from build123d import *

# Parameters (mm, degrees)
SKETCH_1_W       = 50
SKETCH_1_H       = 100
EXTRUDE_1_DEPTH  = 4
FILLET_2_R       = 5
FILLET_3_R       = 5
FILLET_4_R       = 5
FILLET_5_R       = 5
SKETCH_2_R       = 3
EXTRUDE_2_DEPTH  = 10
SKETCH_3_R       = 3
EXTRUDE_3_DEPTH  = 15
SKETCH_6_W       = 50
SKETCH_6_H       = 100
EXTRUDE_4_DEPTH  = 4
FILLET_6_R       = 5
FILLET_7_R       = 5
FILLET_8_R       = 5
FILLET_9_R       = 5
SKETCH_7_W       = 50
SKETCH_7_H       = 100
EXTRUDE_5_DEPTH  = 4
EXTRUDE_START    = 15
SKETCH_8_R       = 3
EXTRUDE_6_DEPTH  = 15
SKETCH_9_W       = 50
SKETCH_9_H       = 100
EXTRUDE_7_DEPTH  = 4
SKETCH_11_R      = 3
EXTRUDE_9_DEPTH  = 15
FILLET_10_R      = 5
FILLET_11_R      = 5
FILLET_12_R      = 5
FILLET_13_R      = 5
FILLET_14_R      = 5
FILLET_15_R      = 5
FILLET_16_R      = 5
FILLET_17_R      = 5
SKETCH_13_W      = 50
SKETCH_13_H      = 100
EXTRUDE_10_DEPTH = 4
SKETCH_14_R      = 3
EXTRUDE_11_DEPTH = 15
FILLET_18_R      = 5
FILLET_19_R      = 5
FILLET_20_R      = 5
FILLET_21_R      = 5
SKETCH_15_R      = 3
EXTRUDE_12_DEPTH = 10
SHELL_1_T        = -0.5


with BuildPart() as part:
    # Sketch 1 → Extrude 1 (new body)
    with BuildSketch(Plane.XY):
        Rectangle(SKETCH_1_W, SKETCH_1_H)
    extrude(amount=EXTRUDE_1_DEPTH)

    # Fillet 2
    fillet_2_edges = [part.edges().sort_by_distance(p)[0] for p in [
        (25, 50, 2),
    ]]
    fillet(fillet_2_edges, radius=FILLET_2_R)

    # Fillet 3
    fillet_3_edges = [part.edges().sort_by_distance(p)[0] for p in [
        (-25, 50, 2),
    ]]
    fillet(fillet_3_edges, radius=FILLET_3_R)

    # Fillet 4
    fillet_4_edges = [part.edges().sort_by_distance(p)[0] for p in [
        (25, -50, 2),
    ]]
    fillet(fillet_4_edges, radius=FILLET_4_R)

    # Fillet 5
    fillet_5_edges = [part.edges().sort_by_distance(p)[0] for p in [
        (-25, -50, 2),
    ]]
    fillet(fillet_5_edges, radius=FILLET_5_R)

    # Sketch 2 → Extrude 2 (add)
    with BuildSketch(Plane.XY.offset(4)):
        with Locations((20, 45)):
            Circle(SKETCH_2_R)
    extrude(amount=EXTRUDE_2_DEPTH)

    # Sketch 3 → Extrude 3 (add)
    with BuildSketch(Plane(origin=(0, 0, 0), x_dir=(-1, 0, 0), z_dir=(0, 0, -1))):
        with Locations(Location((20, -45, 0), (0, 0, 180))):
            Circle(SKETCH_3_R)
    extrude(amount=EXTRUDE_3_DEPTH)

    # Sketch 6 → Extrude 4 (add)
    with BuildSketch(Plane(origin=(0, 0, -15), x_dir=(-1, 0, 0), z_dir=(0, 0, -1))):
        Rectangle(SKETCH_6_W, SKETCH_6_H)
    extrude(amount=EXTRUDE_4_DEPTH)

    # Fillet 6
    fillet_6_edges = [part.edges().sort_by_distance(p)[0] for p in [
        (25, 50, -17),
    ]]
    fillet(fillet_6_edges, radius=FILLET_6_R)

    # Fillet 7
    fillet_7_edges = [part.edges().sort_by_distance(p)[0] for p in [
        (-25, 50, -17),
    ]]
    fillet(fillet_7_edges, radius=FILLET_7_R)

    # Fillet 8
    fillet_8_edges = [part.edges().sort_by_distance(p)[0] for p in [
        (-25, -50, -17),
    ]]
    fillet(fillet_8_edges, radius=FILLET_8_R)

    # Fillet 9
    fillet_9_edges = [part.edges().sort_by_distance(p)[0] for p in [
        (25, -50, -17),
    ]]
    fillet(fillet_9_edges, radius=FILLET_9_R)



with BuildPart() as body_2:
    # Sketch 7 → Extrude 5 (new body)
    with BuildSketch(Plane(origin=(0, 0, -34), x_dir=(-1, 0, 0), z_dir=(0, 0, -1))):
        Rectangle(SKETCH_7_W, SKETCH_7_H)
    extrude(amount=EXTRUDE_5_DEPTH)


with BuildPart() as part_1:
    add(part.part)

    add(body_2.part)  # Extrude 6 merges body 2
    # Sketch 8 → Extrude 6 (add)
    with BuildSketch(Plane(origin=(0, 0, -19), x_dir=(-1, 0, 0), z_dir=(0, 0, -1)).offset(EXTRUDE_START)):
        with Locations(Location((-20, 45, 0), (0, 0, 180))):
            Circle(SKETCH_8_R)
    extrude(amount=-EXTRUDE_6_DEPTH)



with BuildPart() as body_2_2:
    # Sketch 9 → Extrude 7 (new body)
    with BuildSketch(Plane(origin=(0, 0, -53), x_dir=(-1, 0, 0), z_dir=(0, 0, -1))):
        Rectangle(SKETCH_9_W, SKETCH_9_H)
    extrude(amount=EXTRUDE_7_DEPTH)


with BuildPart() as part_2:
    add(part_1.part)

    add(body_2_2.part)  # Extrude 9 merges body 2 2
    # Sketch 11 → Extrude 9 (add)
    with BuildSketch(Plane(origin=(0, 0, -38), x_dir=(-1, 0, 0), z_dir=(0, 0, -1))):
        with Locations(Location((20, -45, 0), (0, 0, 180))):
            Circle(SKETCH_11_R)
    extrude(amount=EXTRUDE_9_DEPTH)

    # Fillet 10
    fillet_10_edges = [part_2.edges().sort_by_distance(p)[0] for p in [
        (25, 50, -36),
    ]]
    fillet(fillet_10_edges, radius=FILLET_10_R)

    # Fillet 11
    fillet_11_edges = [part_2.edges().sort_by_distance(p)[0] for p in [
        (25, 50, -55),
    ]]
    fillet(fillet_11_edges, radius=FILLET_11_R)

    # Fillet 12
    fillet_12_edges = [part_2.edges().sort_by_distance(p)[0] for p in [
        (-25, 50, -55),
    ]]
    fillet(fillet_12_edges, radius=FILLET_12_R)

    # Fillet 13
    fillet_13_edges = [part_2.edges().sort_by_distance(p)[0] for p in [
        (-25, 50, -36),
    ]]
    fillet(fillet_13_edges, radius=FILLET_13_R)

    # Fillet 14
    fillet_14_edges = [part_2.edges().sort_by_distance(p)[0] for p in [
        (-25, -50, -55),
    ]]
    fillet(fillet_14_edges, radius=FILLET_14_R)

    # Fillet 15
    fillet_15_edges = [part_2.edges().sort_by_distance(p)[0] for p in [
        (-25, -50, -36),
    ]]
    fillet(fillet_15_edges, radius=FILLET_15_R)

    # Fillet 16
    fillet_16_edges = [part_2.edges().sort_by_distance(p)[0] for p in [
        (25, -50, -55),
    ]]
    fillet(fillet_16_edges, radius=FILLET_16_R)

    # Fillet 17
    fillet_17_edges = [part_2.edges().sort_by_distance(p)[0] for p in [
        (25, -50, -36),
    ]]
    fillet(fillet_17_edges, radius=FILLET_17_R)



with BuildPart() as body_2_3:
    # Sketch 13 → Extrude 10 (new body)
    with BuildSketch(Plane(origin=(0, 0, -72), x_dir=(-1, 0, 0), z_dir=(0, 0, -1))):
        Rectangle(SKETCH_13_W, SKETCH_13_H)
    extrude(amount=EXTRUDE_10_DEPTH)


with BuildPart() as part_3:
    add(part_2.part)

    add(body_2_3.part)  # Extrude 11 merges body 2 3
    # Sketch 14 → Extrude 11 (add)
    with BuildSketch(Plane(origin=(0, 0, -57), x_dir=(-1, 0, 0), z_dir=(0, 0, -1)).offset(EXTRUDE_START)):
        with Locations(Location((-20, 45, 0), (0, 0, 180))):
            Circle(SKETCH_14_R)
    extrude(amount=-EXTRUDE_11_DEPTH)

    # Fillet 18
    fillet_18_edges = [part_3.edges().sort_by_distance(p)[0] for p in [
        (25, 50, -74),
    ]]
    fillet(fillet_18_edges, radius=FILLET_18_R)

    # Fillet 19
    fillet_19_edges = [part_3.edges().sort_by_distance(p)[0] for p in [
        (-25, 50, -74),
    ]]
    fillet(fillet_19_edges, radius=FILLET_19_R)

    # Fillet 20
    fillet_20_edges = [part_3.edges().sort_by_distance(p)[0] for p in [
        (25, -50, -74),
    ]]
    fillet(fillet_20_edges, radius=FILLET_20_R)

    # Fillet 21
    fillet_21_edges = [part_3.edges().sort_by_distance(p)[0] for p in [
        (-25, -50, -74),
    ]]
    fillet(fillet_21_edges, radius=FILLET_21_R)

    # Sketch 15 → Extrude 12 (add)
    with BuildSketch(Plane(origin=(0, 0, -76), x_dir=(-1, 0, 0), z_dir=(0, 0, -1))):
        with Locations(Location((20, -45, 0), (0, 0, 180))):
            Circle(SKETCH_15_R)
    extrude(amount=EXTRUDE_12_DEPTH)

    # Shell 1
    shell_1_openings = [part_3.faces().sort_by_distance(p)[0] for p in [
        (-20, -45, -86),
        (20, 45, 14),
    ]]
    offset(amount=SHELL_1_T, openings=shell_1_openings, kind=Kind.INTERSECTION)


solid = part_3.part
Source: CAD feature listing. Evaluate the final solid. Frame: model axes, mm. A direction names the side the tool comes from. Coordinates: 2 decimals unless noted, no trailing zeros. Loops run counter-clockwise (first coordinate to the right, second up) from the corner with the lowest first, then second, coordinate; pieces in that order, holes last. Notation, with made-up numbers: (2, 10) - (32, 10) arc R24 ccw to (32, 29) - close; hole circle Ø11 at (69.25, 72.25). An arc over 180 degrees is marked (long way). One line per item, written item: value. Start each with the question number.
1. Ray query, L1, parallel to Y at x = -20, z = -11; L2, parallel to X at y = -3, z = -73; L3, parallel to X at y = 45, z = -25.75. Return the intervals inside material, ascending.
2. Contact query for flat-ended pins moving along their axis: P1, Ø3, axis at x = -20, y = -45, coming from the +Z side; P2, Ø5, axis at x = 2.5, y = 0.5, coming from the -Z side; P3, Ø1.5, axis at y = 32.5, z = -14, coming from the -X side. Output: stop coordinate, or through.
3. Mould query, pull axis Y, two halves, no side actions, for faces 1 (the flat face through (-24.5, -1, -55)), 2 (the cylindrical face through (24, 48, 2)), 3 (the flat face through (25, -1, -36)). Classes: pulls with the +Y half, pulls with the -Y half, needs draft (parallel to the pull), parting line crosses it, or undercut.
4. Section C-C (z = -13.5). Return the cut outline in (x, y), and give its area (3 significant figures).
5. Section A-A (y = 3). State how many separate pieces and enclosed holes the cut face has, and give its area (3 significant figures).
6. Set-up query: faces 4 (the flat face through (0, 49.5, -36)), 5 (the flat face through (25, -1, -17)). Return all of +Z, -Z, +X, -X, +Y, -Y with unobstructed straight access to the full face (end or side cutting, diameter ignored); none if empty.
Verdict:
1. L1: y = -48 to -47.5, -42.5 to -42
1. L2: x = -25 to -24.5, 24.5 to 25
1. L3: x = 17 to 17.5, 22.5 to 23
2. P1: stops at z = 4
2. P2: stops at z = -76
2. P3: passes through
3. face 1: undercut
3. face 2: pulls with the +Y half
3. face 3: needs draft
4. outline: circle Ø6 at (-20, -45); hole circle Ø5 at (-20, -45)
4. area: 8.64 mm2
5. separate pieces: 5
5. enclosed holes: 5
5. area: 265 mm2
6. face 4: none
6. face 5: +Z, -Z, +X, +Y, -Y
